Build history of the part. All positions in model axes, mm. A direction names the side the tool comes from. Round coordinates to 2 decimals unless told otherwise and drop trailing zeros. Write each loop counter-clockwise with the first axis right and the second up, starting at its lowest first coordinate (ties: lowest second). Pieces come first, ordered by that corner, then holes.
1) Saw through at B-B (x = -7). Write the cut outline in (y, z), plus the area to 3 significant figures.
2) Saw through at C-C (z = 0). Write the cut outline in (x, y).
3) Wall check: probe 1 along Z at (x, y) = (-2.5, -24); probe 2 along X at (y, z) = (-8.5, 2). Give the ranges that are in metal, low to high.
4) Flat gauge pins, fed straight in: pin 1 (5 mm diameter, centred on x = 39, y = 11, fed in from -Z); pin 2 (2.5 mm diameter, centred on x = 11, z = 6.5, fed in from +Y); pin 3 (6.5 mm diameter, centred on y = -25, z = 1.5, fed in from -X); pin 4 (10 mm diameter, centred on y = 23, z = 37, fed in from +X). Where does each tip first touch, or does it go through?
5) Which spindle directions (+Z, -Z, +X, -X, +Y, -Y) get a long thin tool onto all of the face, cutting with end or side? Do faces 1 (the flat face through (-50, 0, 12.5)), 2 (the flat face through (-65, 0, 64)), 3 (the flat face through (0, -25, -8)), 4 (the flat face through (-1, 20.32, 15)), 5 (the flat face through (-65, -17.32, 64)). Say none if no direction does.
6) Saw through at A-A (z = 23.5). Write the cut outline in (x, y).
7) Pull direction Y, two halves, no side cores. Call faces 6 (the flat face through (0, -25, 8)), 7 (the flat face through (30.5, -25, 0)), 8 (the flat face through (25, 0, 0)): +Y half, -Y half, draft (parallel to the pull), parting line (faces both ways), or undercut.
Autodesk Inventor part; units mm, degrees
ref_plane "YZ Plane" through (0, 0, 0) normal (1, 0, 0) x (0, 1, 0)
ref_plane "XZ Plane" through (0, 0, 0) normal (0, 1, 0) x (-1, 0, 0)
ref_plane "XY Plane" through (0, 0, 0) normal (0, 0, 1) x (1, 0, 0)
sketch "Esquisse1" plane through (0, 0, 0) normal (1, 0, 0) x (0, 1, 0)
  line L0 (25, -12.5) -> (-25, -12.5)
  line L1 (-25, -12.5) -> (-25, 12.5)
  line L2 (-25, 12.5) -> (25, 12.5)
  line L3 (25, 12.5) -> (25, -12.5)
  line L4 (25, -12.5) -> (-25, 12.5) construction
  line L5 (-25, -12.5) -> (25, 12.5) construction
  circle A0 centre (25, 0) radius 12.5
  circle A1 centre (25, 0) radius 4
  circle A2 centre (-25, 0) radius 4
  circle A3 centre (-25, 0) radius 12.5
  point P0 (0, 0)
  point P1 (-25, -12.5)
  point P2 (25, -12.5)
  point P3 (25, -4)
  point P4 (25, 4)
  point P5 (-25, 4)
  point P6 (-25, -4)
  dimension "d1" = 25
  dimension "d0" = 8
  dimension "d2" = 50
extrude "Extrusion1" add sketch "Esquisse1" along normal mid plane 61 contours A1 L3 | L3 A1 | A2 L1 | L1 A2
extrude "Extrusion2" add sketch "Esquisse1" along normal mid plane 50 contours A0 L3 A1 | L0 A3 L2 A0 | L1 A2 A3 picked at (24.0029, -9.5456) picked at (-15.4378, -0.9272)
sketch "Esquisse2" plane through (-25, -25, 12.5) normal (0, 0, 1) x (1, 0, 0)
  line L0 (0, 0) -> (0, 50)
  line L1 (50, 50) -> (50, 0)
  line L2 (0, 0) -> (50, 0)
  line L3 (-50, 7.6795) -> (-30, 7.6795)
  line L4 (-30, 7.6795) -> (25, 7.6795)
  line L5 (25, 7.6795) -> (80, 7.6795)
  line L6 (80, 7.6795) -> (100, 7.6795)
  line L7 (100, 7.6795) -> (100, 42.3205)
  line L8 (100, 42.3205) -> (80, 7.6795)
  line L9 (-30, 7.6795) -> (-50, 42.3205)
  line L10 (-50, 42.3205) -> (-50, 7.6795)
  line L11 (25, -15.6) -> (25, 65.6)
  line L12 (-50, 45.3205) -> (100, 45.3205)
  line L13 (100, 45.3205) -> (100, 4.6795)
  line L14 (100, 4.6795) -> (-50, 4.6795)
  line L15 (-50, 4.6795) -> (-50, 45.3205)
  line L16 (-50, 42.3205) -> (-50, 45.3205) construction
  line L17 (-50, 7.6795) -> (-50, 4.6795) construction
  line L18 (100, 42.3205) -> (100, 45.3205) construction
  line L19 (100, 7.6795) -> (100, 4.6795) construction
  line L20 (-50, 4.6795) -> (25, 25) construction
  line L21 (25, 25) -> (100, 45.3205) construction
  dimension "d14" = 34.641
  dimension "d15" = 110
  dimension "d16" = 20
  dimension "d17" = 17.3205
  dimension "d18" = 60
  dimension "d22" = 3
extrude "Extrusion3" add sketch "Esquisse2" along normal blind 100 contours L3 L10 L9 | L8 L7 L6
extrude "Extrusion4" add sketch "Esquisse2" along normal blind 5 contours L14 L15 L3 L4 L0 | L0 L4 L11 L14 | L4 L9 L15 L12 L0 | L0 L12 L11 L4 | L11 L5 L1 L14 | L3 L10 L9 | L11 L12 L1 L5 | L1 L5 L6 L13 L14 | L1 L12 L13 L8 L5 | L8 L7 L6
properties part number "Doigt trans"
Evaluation:
1. outline: (-25, -12.5) - (25, -12.5) - (25, -4) arc R4 ccw to (25, 4) - (25, 12.5) - (20.32, 12.5) - (20.32, 17.5) - (-20.32, 17.5) - (-20.32, 12.5) - (-25, 12.5) - (-25, 4) arc R4 ccw to (-25, -4) - close
1. area: 1,500 mm2
2. outline: (-30.5, -29) - (30.5, -29) - (30.5, -21) - (25, -21) - (25, 21) - (30.5, 21) - (30.5, 29) - (-30.5, 29) - (-30.5, 21) - (-25, 21) - (-25, -21) - (-30.5, -21) - close
3. probe 1: z = -12.5 to 12.5
3. probe 2: x = -25 to 25
4. pin 1: stops at z = 12.5
4. pin 2: stops at y = 25
4. pin 3: stops at x = -30.5
4. pin 4: passes through
5. face 1: -Z, -X, +Y, -Y
5. face 2: +Z, +Y
5. face 3: -Z, +X, -X, -Y
5. face 4: +Z, +X, -X, +Y
5. face 5: +Z, +X, -X, -Y
6. outline: (-75, -17.32) - (-55, -17.32) - (-75, 17.32) - close; (55, -17.32) - (75, -17.32) - (75, 17.32) - close
7. face 6: -Y half
7. face 7: draft
7. face 8: undercut
